Verification items for the finished model (mm, model axes). Coordinates: 2 decimals unless noted, no trailing zeros. Order: outer loops, then holes, each group sorted by start corner. A loop starts at its lowest first (then second) coordinate and runs counter-clockwise, first axis right, second up.
Q1. Thickness scan on line 1 (Y direction, x = 0.75, z = -88); line 2 (X direction, y = -8.25, z = 89); line 3 (Y direction, x = -6.25, z = -7). Record the ranges inside material, lowest first.
Q2. Depth check by flat-ended pin: P1, Ø1.6, axis at y = 0.5, z = 2.5, coming from the +X side; P2, Ø2.5, axis at x = -0.5, z = 27, coming from the +Y side; P3, Ø2.5, axis at x = -0.5, z = 43.5, coming from the -Y side. Enter the tip coordinate at first touch or a pass-through.
Q3. Cross-section at A-A, the plane y = 0. Record the boundary of the cut face in (x, z), and give its area (3 significant figures).
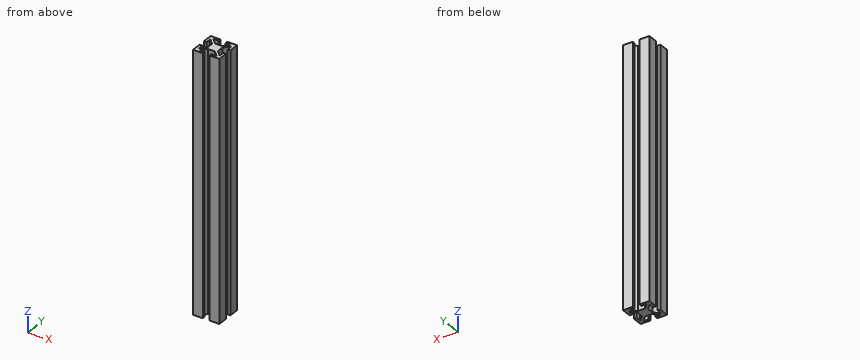
from build123d import *

# Parameters (mm, degrees)
BOSS_EXTRUDE1_DEPTH = 98
SKETCH2_R           = 2.5
CUT_EXTRUDE1_DEPTH  = 10


with BuildPart() as part:
    # Sketch1 → Boss-Extrude1 (new body, symmetric)
    with BuildSketch(Plane.XY):
        Polygon((-2.585786438, 4), (2.585786438, 4), (6.585786438, 8), (2.5, 8), (2.5, 10), (10, 10), (10, 2.5), (8, 2.5), (8, 6.585786438), (4, 2.585786438), (4, -2.585786438), (8, -6.585786438), (8, -2.5), (10, -2.5), (10, -10), (2.5, -10), (2.5, -8), (6.585786438, -8), (2.585786438, -4), (-2.585786438, -4), (-6.585786438, -8), (-2.5, -8), (-2.5, -10), (-10, -10), (-10, -2.5), (-8, -2.5), (-8, -6.585786438), (-4, -2.585786438), (-4, 2.585786438), (-8, 6.585786438), (-8, 2.5), (-10, 2.5), (-10, 10), (-2.5, 10), (-2.5, 8), (-6.585786438, 8), align=None)
    extrude(amount=BOSS_EXTRUDE1_DEPTH, both=True)

    # Sketch2 → Cut-Extrude1 (cut)
    with BuildSketch(Plane(origin=(4, 0, 0), x_dir=(0, 0, -1), z_dir=(1, 0, 0))):
        with Locations((88, 0)):
            Circle(SKETCH2_R)
    extrude(amount=-CUT_EXTRUDE1_DEPTH, mode=Mode.SUBTRACT)


solid = part.part
Check values:
1. line 1: y = -4 to -2.5, 2.5 to 4
1. line 2: x = -10 to -2.5, 2.5 to 10
1. line 3: y = -10 to -8, -7.66 to -4.84, 4.84 to 7.66, 8 to 10
2. P1: stops at x = 4
2. P2: stops at y = 4
2. P3: stops at y = -4
3. outline: (-4, -98) - (4, -98) - (4, -90.5) - (-4, -90.5) - close; (-4, -85.5) - (4, -85.5) - (4, 98) - (-4, 98) - close
3. area: 1,530 mm2
